Can you work these out from the drawing? Everything is in mm from the part's minimum corner. A direction names the side the tool comes from. Give positions to 0.01 mm unless a question says otherwise; leave off trailing zeros. Write each loop counter-clockwise with the first axis right and the second up, starting at its lowest first coordinate (ties: lowest second). Pieces come first, ordered by that corner, then holes. Notation, with made-up numbers: (-2.5, 67) - (8.5, 67) arc R19 cw to (8.5, 103) - close; hole circle Ø3 at (22, 3). An arc over 180 degrees is marked (long way). Answer in a Markdown table with one row per item.
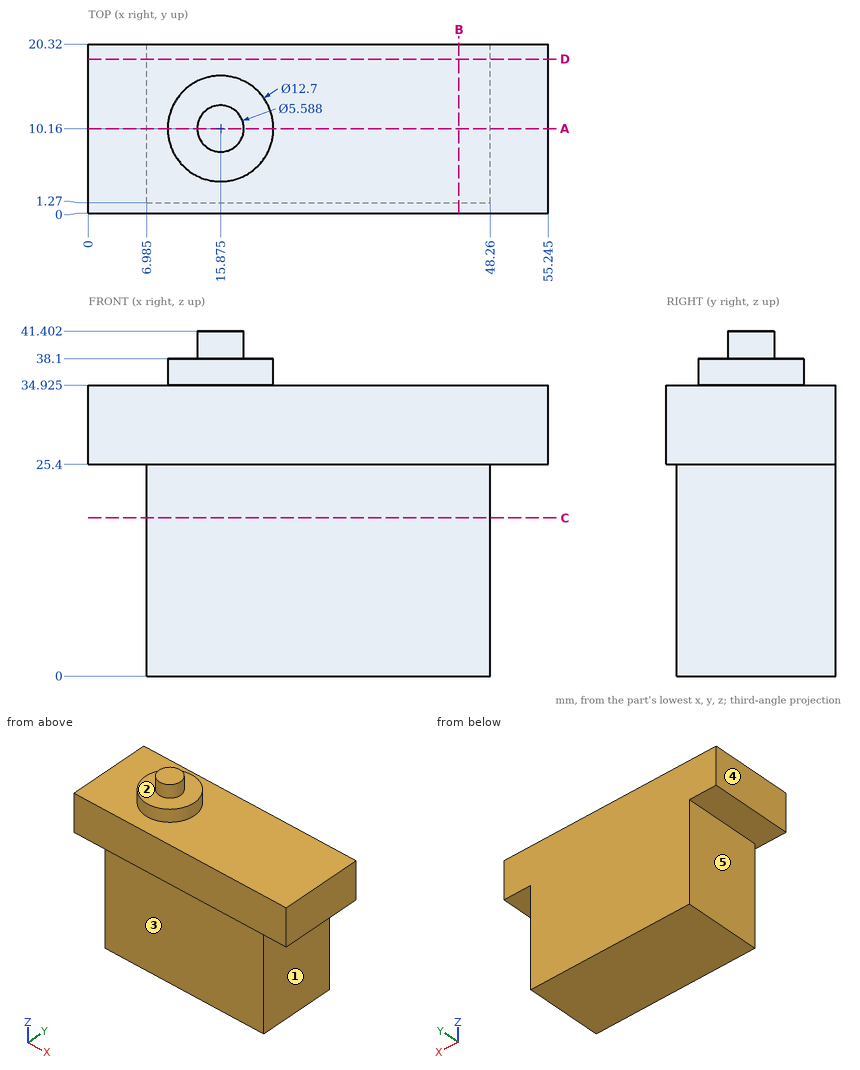
1) Imagine slicing it at C-C (z = 19). List the corners of the cut face in (x, y) for me (3 decimals), then the cut area to 3 significant figures.
Check values:
| item | result |
|---|---|
| outline | (6.985, 1.27) - (48.26, 1.27) - (48.26, 20.32) - (6.985, 20.32) - close |
| area | 786 mm2 |
2) Imagine slicing it at A-A (y = 10.16). List the corners of the cut face in (x, z) for me (3 decimals).
Check values:
| item | result |
|---|---|
| outline | (0, 25.4) - (6.985, 25.4) - (6.985, 0) - (48.26, 0) - (48.26, 25.4) - (55.245, 25.4) - (55.245, 34.925) - (22.225, 34.925) - (22.225, 38.1) - (18.669, 38.1) - (18.669, 41.402) - (13.081, 41.402) - (13.081, 38.1) - (9.525, 38.1) - (9.525, 34.925) - (0, 34.925) - close |
3) Imagine slicing it at B-B (x = 44.5). List the corners of the cut face in (y, z) for me (3 decimals), then the cut area to 3 significant figures.
Check values:
| item | result |
|---|---|
| outline | (0, 25.4) - (1.27, 25.4) - (1.27, 0) - (20.32, 0) - (20.32, 34.925) - (0, 34.925) - close |
| area | 677 mm2 |
4) If I drill on line 1 (X direction, y = 16, z = 3) (3 decimals); line 2 (Z direction, x = 10, y = 17) (3 decimals); line 3 (Y direction, x = 25.5, z = 13.5), over which ranges is the centre line in solid material (lowest first)?
Check values:
| item | result |
|---|---|
| line 1 | x = 6.985 to 48.26 |
| line 2 | z = 0 to 34.925 |
| line 3 | y = 1.27 to 20.32 |
5) Will these pins go through, and if not, where does the flat tip stop? P1, Ø1.5, axis at x = 14, z = 29.5, coming from the -Y side; P2, Ø6, axis at y = 8, z = 15, coming from the -X side (3 decimals); P3, Ø8, axis at x = 41, z = 14, coming from the -Y side.
Check values:
| item | result |
|---|---|
| P1 | stops at y = 0 |
| P2 | stops at x = 6.985 |
| P3 | stops at y = 1.27 |
6) On a 3-axis mill with a long thin cutter (end or side, diameter ignored), from which of +Z, -Z, +X, -X, +Y, -Y can I reach the whole of each face in a straight line? I mean the marked faces 1, 2, 3, 4 and 5. Say none if no direction works.
Check values:
| item | result |
|---|---|
| face 1 | -Z, +X, +Y, -Y |
| face 2 | +Z |
| face 3 | -Z, +X, -X, -Y |
| face 4 | +Z, -Z, -X, +Y, -Y |
| face 5 | -Z, -X, +Y, -Y |
7) Imagine slicing it at D-D (y = 18.5). List the corners of the cut face in (x, z) for me (3 decimals), then the cut area to 3 significant figures.
Check values:
| item | result |
|---|---|
| outline | (0, 25.4) - (6.985, 25.4) - (6.985, 0) - (48.26, 0) - (48.26, 25.4) - (55.245, 25.4) - (55.245, 34.925) - (0, 34.925) - close |
| area | 1,570 mm2 |
